from build123d import *

# Parameters (mm, degrees)
BOSS_EXTRUDE1_DEPTH   = 5
SKETCH1_R             = 2
BOSS_EXTRUDE1_2_DEPTH = 5
BOSS_EXTRUDE1_3_DEPTH = 5
BOSS_EXTRUDE1_4_DEPTH = 5
BOSS_EXTRUDE1_5_DEPTH = 5
SKETCH1_3_W           = 20
SKETCH1_3_H           = 20
BOSS_EXTRUDE2_DEPTH   = 2


with BuildPart() as part:
    # Sketch1 → Boss-Extrude1 (new body)
    with BuildSketch(Plane.XY):
        Polygon((4.925, 10), (-4.925, 10), (-3.125, 8.2), (-5.5, 8.2), (-5.5, 6.560660172), (-2.839339828, 3.9), (2.839339828, 3.9), (5.5, 6.560660172), (5.5, 8.2), (3.125, 8.2), align=None)
    extrude(amount=BOSS_EXTRUDE1_DEPTH)



with BuildPart() as body_2:
    # Sketch1 → Boss-Extrude1 2 (new body)
    with BuildSketch(Plane.XY):
        Circle(SKETCH1_R)
    extrude(amount=BOSS_EXTRUDE1_2_DEPTH)


with BuildPart() as body_3:
    # Sketch1 → Boss-Extrude1 3 (new body)
    with BuildSketch(Plane.XY):
        Polygon((10, -4.925), (10, 4.925), (8.2, 3.125), (8.2, 5.5), (6.560660172, 5.5), (3.9, 2.839339828), (3.9, -2.839339828), (6.560660172, -5.5), (8.2, -5.5), (8.2, -3.125), align=None)
    extrude(amount=BOSS_EXTRUDE1_3_DEPTH)


with BuildPart() as body_4:
    # Sketch1 → Boss-Extrude1 4 (new body)
    with BuildSketch(Plane.XY):
        Polygon((-8.2, 3.125), (-10, 4.925), (-10, -4.925), (-8.2, -3.125), (-8.2, -5.5), (-6.560660172, -5.5), (-3.9, -2.839339828), (-3.9, 2.839339828), (-6.560660172, 5.5), (-8.2, 5.5), align=None)
    extrude(amount=BOSS_EXTRUDE1_4_DEPTH)


with BuildPart() as body_5:
    # Sketch1 → Boss-Extrude1 5 (new body)
    with BuildSketch(Plane.XY):
        Polygon((-3.125, -8.2), (-4.925, -10), (4.925, -10), (3.125, -8.2), (5.5, -8.2), (5.5, -6.560660172), (2.839339828, -3.9), (-2.839339828, -3.9), (-5.5, -6.560660172), (-5.5, -8.2), align=None)
    extrude(amount=BOSS_EXTRUDE1_5_DEPTH)


with BuildPart() as part_1:
    add(part.part)

    add(body_2.part)  # Boss-Extrude2 merges body 2

    add(body_3.part)  # Boss-Extrude2 merges body 3

    add(body_4.part)  # Boss-Extrude2 merges body 4

    add(body_5.part)  # Boss-Extrude2 merges body 5
    # Sketch1<3> → Boss-Extrude2 (add)
    with BuildSketch(Plane.XY):
        Rectangle(SKETCH1_3_W, SKETCH1_3_H)
    extrude(amount=-BOSS_EXTRUDE2_DEPTH)


solid = part_1.part
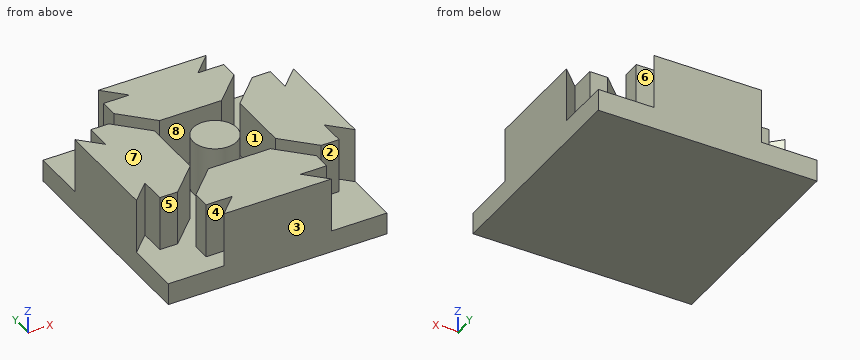
Could you check a few things on this model? Use its own coordinates, in mm. Face numbers are marked on the shaded views. A direction names the side the tool comes from. Coordinates: 2 decimals unless noted, no trailing zeros. Loops run counter-clockwise (first coordinate to the right, second up) from the corner with the lowest first, then second, coordinate; pieces in that order, holes last.
1. Imagine slicing it at B-B (y = 0). Please give me the cut outline in (x, z), and give its area (3 significant figures).
2. Imagine slicing it at C-C (z = 4). Give the number of separate pieces and of enclosed holes in the cut face, and give its area (3 significant figures).
3. For P1, Ø1, axis at y = 8, z = 3.5, coming from the -X side; P2, Ø1.3, axis at x = 7.5, z = 2, coming from the +Y side; P3, Ø0.8, axis at x = 7.5, z = 2.5, coming from the -Y side, each with a flat end and sliding along its axis, tell me the tip position at first contact or that it passes through.
4. Imagine slicing it at A-A (x = -7.25). Please give me the cut outline in (y, z).
5. We'd pull the mould along Y, two halves only. Please class the marked faces 5, 6, 7 and 8: released by +Y, released by -Y, zero draft, split by the parting line, or undercut.
6. I need wall thicknesses on L1, parallel to Y at x = -3.5, z = 1.5 (3 decimals); L2, parallel to Y at x = -1.5, z = 1; L3, parallel to Y at x = -1, z = 1.75. Which ranges of each line are inside material? Lowest first, please.
7. For the marked faces 1, 2, 3 and 4, which set-ups out of +Z, -Z, +X, -X, +Y, -Y let a thin tool reach every point of the face, with its end or its side?
Computed values:
1. outline: (-10, -2) - (10, -2) - (10, 5) - (3.9, 5) - (3.9, 0) - (2, 0) - (2, 5) - (-2, 5) - (-2, 0) - (-3.9, 0) - (-3.9, 5) - (-10, 5) - close
1. area: 121 mm2
2. separate pieces: 5
2. enclosed holes: 0
2. area: 231 mm2
3. P1: stops at x = -5.5
3. P2: stops at y = 5.5
3. P3: stops at y = -5.5
4. outline: (-10, -2) - (10, -2) - (10, 0) - (5.5, 0) - (5.5, 5) - (-5.5, 5) - (-5.5, 0) - (-10, 0) - close
5. face 5: released by -Y
5. face 6: undercut
5. face 7: zero draft
5. face 8: undercut
6. L1: y = -10 to -8.575, -8.2 to -4.561, 4.561 to 8.2, 8.575 to 10
6. L2: y = -10 to -3.9, -1.32 to 1.32, 3.9 to 10
6. L3: y = -10 to -3.9, -1.73 to 1.73, 3.9 to 10
7. face 1: +Z
7. face 2: +Z, +X, -Y
7. face 3: +Z, -Z, +X, -X, -Y
7. face 4: +Z, -X
